Check sheet for the drawn part. Datum: minimum x, y, z corner. Units: mm. Round coordinates to 2 decimals unless told otherwise and drop trailing zeros. Loops run counter-clockwise (first coordinate to the right, second up) from the corner with the lowest first, then second, coordinate; pieces in that order, holes last.
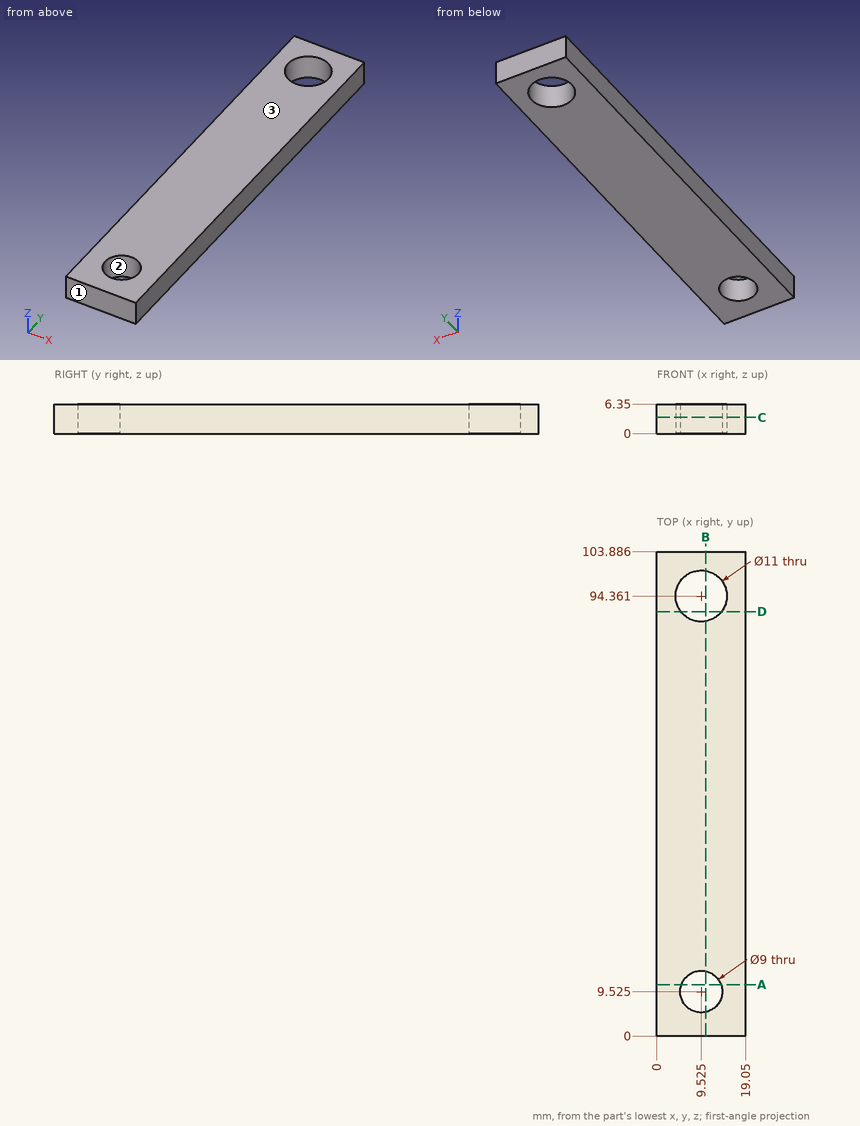
1. Section check C-C (z = 3.5). Enter the section's corners in (x, y) (3 decimals), then the cut area to 3 significant figures.
2. Gauge pin test, flat end, axial feed: P1, Ø3, axis at y = 32, z = 4, coming from the -X side. Record the tip position at first contact, or that the pin passes through.
3. Scan lines: L1, parallel to Y at x = 9.5, z = 5.5; L2, parallel to Y at x = 5.5, z = 4.5; L3, parallel to X at y = 92.5, z = 2.75. Record each from-to range of solid material in increasing order.
4. Section check D-D (y = 91). Enter the section's corners in (x, z), then the cut area to 3 significant figures.
5. Section check B-B (x = 10.5). Enter the section's corners in (y, z).
6. Release check for a two-part mould opening along Y. For the marked faces 1, 2 and 3 record: released by +Y, released by -Y, zero draft, split by the parting line, or undercut.
7. Section check A-A (y = 11). Enter the section's corners in (x, z).
Taken from the geometry:
1. outline: (0, 0) - (19.05, 0) - (19.05, 103.886) - (0, 103.886) - close; hole circle Ø11 at (9.525, 94.361); hole circle Ø9 at (9.525, 9.525)
1. area: 1,820 mm2
2. P1: stops at x = 0
3. L1: y = 0 to 5.03, 14.02 to 88.86, 99.86 to 103.89
3. L2: y = 0 to 7.51, 11.54 to 90.61, 98.11 to 103.89
3. L3: x = 0 to 4.35, 14.7 to 19.05
4. outline: (0, 0) - (5.17, 0) - (5.17, 6.35) - (0, 6.35) - close; (13.88, 0) - (19.05, 0) - (19.05, 6.35) - (13.88, 6.35) - close
4. area: 65.7 mm2
5. outline: (0, 0) - (5.13, 0) - (5.13, 6.35) - (0, 6.35) - close; (13.92, 0) - (88.95, 0) - (88.95, 6.35) - (13.92, 6.35) - close; (99.77, 0) - (103.89, 0) - (103.89, 6.35) - (99.77, 6.35) - close
6. face 1: released by -Y
6. face 2: undercut
6. face 3: zero draft
7. outline: (0, 0) - (5.27, 0) - (5.27, 6.35) - (0, 6.35) - close; (13.78, 0) - (19.05, 0) - (19.05, 6.35) - (13.78, 6.35) - close
